```python
from build123d import *

# Parameters (mm, degrees)
SKETCH_1_R          = 1.35
SKETCH_1_R_2        = 1
EXTRUDE_1_DEPTH     = 3
SKETCH_2_R          = 1.6
CUT_EXTRUDE_1_DEPTH = 37.133094234


with BuildPart() as part:
    # 草图1 → 凸台-拉伸1 (new body)
    with BuildSketch(Plane.XY.offset(3)):
        with BuildLine():
            Line((13.843681844, 23.9998), (-3.157118156, 23.9998))
            ThreePointArc((-3.157118156, 23.9998), (-5.2784385, 23.121120344), (-6.157118156, 20.9998))
            Line((-6.157118156, 20.9998), (-6.157118156, 3))
            ThreePointArc((-6.157118156, 3), (-5.2784385, 0.878679656), (-3.157118156, 0))
            Line((-3.157118156, 0), (13.843681844, 0))
            Line((13.843681844, 0), (24.001386189, 0.533010723))
            ThreePointArc((24.001386189, 0.533010723), (26.020372671, 1.463896655), (26.844181844, 3.528889024))
            Line((26.844181844, 3.528889024), (26.844181844, 20.471910982))
            ThreePointArc((26.844181844, 20.471910982), (26.020271299, 22.537010177), (24.001092054, 23.467804703))
            Line((24.001092054, 23.467804703), (13.843681844, 23.9998))
        make_face()
        with Locations(Location((24.044031844, 3.501148349, 0), (0, 0, 180))):
            Circle(SKETCH_1_R, mode=Mode.SUBTRACT)
        with Locations(Location((-3.156018156, 3.501148349, 0), (0, 0, 180))):
            Circle(SKETCH_1_R, mode=Mode.SUBTRACT)
        with Locations(Location((24.044031844, 20.498351651, 0), (0, 0, 180))):
            Circle(SKETCH_1_R, mode=Mode.SUBTRACT)
        with Locations(Location((-3.156018156, 20.498351651, 0), (0, 0, 180))):
            Circle(SKETCH_1_R_2, mode=Mode.SUBTRACT)
        Polygon((21.843181844, 14.4995), (23.343481844, 14.4995), (23.343481844, 9.5), (21.843181844, 9.5), (21.843181844, 6), (16.343381844, 6), (16.343381844, 3), (4.343381844, 3), (4.343381844, 6), (-1.156518156, 6), (-1.156518156, 9.5), (-2.656818156, 9.5), (-2.656818156, 14.4995), (-1.156518156, 14.4995), (-1.156518156, 17.9998), (4.343381844, 17.9998), (4.343381844, 20.9998), (16.343381844, 20.9998), (16.343381844, 17.9998), (21.843181844, 17.9998), align=None, mode=Mode.SUBTRACT)
    extrude(amount=-EXTRUDE_1_DEPTH)

    # 草图2 → 切除-拉伸1 (cut, through all)
    with BuildSketch(Plane.XY.offset(3)):
        with Locations((-3.156018156, 20.498351651)):
            Circle(SKETCH_2_R)
        with Locations((24.044031844, 20.498351651)):
            Circle(SKETCH_2_R)
        with Locations((24.044031844, 3.501148349)):
            Circle(SKETCH_2_R)
        with Locations((-3.156018156, 3.501148349)):
            Circle(SKETCH_2_R)
    extrude(amount=-CUT_EXTRUDE_1_DEPTH, mode=Mode.SUBTRACT)


solid = part.part
```
For this review, take the finished solid that the model builds, in its own axes (mm). A direction names the side the tool comes from. Round coordinates to 2 decimals unless told otherwise and drop trailing zeros. Write each loop counter-clockwise with the first axis right and the second up, starting at its lowest first coordinate (ties: lowest second). Pieces come first, ordered by that corner, then holes. Notation, with made-up numbers: (71.25, 8) - (92.25, 8) arc R17 ccw to (92.25, 16) - close; hole circle Ø2 at (70.25, -38). An arc over 180 degrees is marked (long way). Answer as a JSON object with one key per item and string values.
1. We need section C-C on x = 24.5. Give the boundary of the cut face in (y, z).
Response values:
{"outline": "(0.6, 0) - (1.97, 0) - (1.97, 3) - (0.6, 3) - close; (5.03, 0) - (18.96, 0) - (18.96, 3) - (5.03, 3) - close; (22.03, 0) - (23.4, 0) - (23.4, 3) - (22.03, 3) - close"}
2. We need section B-B on y = 12.25. Give the boundary of the cut face in (x, z).
Response values:
{"outline": "(-6.16, 0) - (-2.66, 0) - (-2.66, 3) - (-6.16, 3) - close; (23.34, 0) - (26.84, 0) - (26.84, 3) - (23.34, 3) - close"}
3. Draft analysis for pull direction X (two halves, no side actions). For faces 3 (the face through (10, 23, 0)), 4 (the face through (25.522, 2.888, 1.521)), 5 (the face through (26, 1.44, 1.52)), state which applies: +X half, -X half, draft (parallel to the pull), parting line (faces both ways), or undercut.
Response values:
{"face 3": "draft", "face 4": "undercut", "face 5": "+X half"}
4. Tool access review of faces 1 (the face through (-2, 14.5, 2)), 2 (the face through (18.851, 0.263, 1.521)): name each direction out of +Z, -Z, +X, -X, +Y, -Y from which nothing blocks a thin tool from reaching the whole face with its end or side.
Response values:
{"face 1": "+Z, -Z", "face 2": "+Z, -Z, +X, -Y"}
5. We need section A-A on x = 1.5. Give the boundary of the cut face in (y, z), then the cut area to 3 significant figures.
Response values:
{"outline": "(0, 0) - (6, 0) - (6, 3) - (0, 3) - close; (18, 0) - (24, 0) - (24, 3) - (18, 3) - close", "area": "36.0 mm2"}
6. For pin 1 Ø1 at (x, z) = (23.5, 0.5) entering from -Y, flat-tipped, find the tip position at first contact; note if it passes through.
Response values:
{"pin 1": "stops at y = 0.48"}
7. We need section D-D on z = 0.95. Count the separate pieces of the cut face and the enclosed holes in it, then the cut area to 3 significant figures.
Response values:
{"separate pieces": "1", "enclosed holes": "5", "area": "381 mm2"}
8. To check wall thickness, follow line 1 along Y through (x, z) = (-3, 2.7); line 2 along X through (y, z) = (13, 0.3); line 3 along Y through (x, z) = (0.5, 1.7). State the ranges of each line that lie inside material, in increasing order.
Response values:
{"line 1": "y = 0 to 1.91, 5.09 to 18.91, 22.09 to 24", "line 2": "x = -6.16 to -2.66, 23.34 to 26.84", "line 3": "y = 0 to 6, 18 to 24"}
